Read the model definition and answer for the solid it produces. Units are mm, in the model's axes. A direction names the side the tool comes from. Give positions to 0.01 mm unless a question says otherwise; leave off trailing zeros. Order: outer loops, then holes, each group sorted by start corner. A loop starts at its lowest first (then second) coordinate and runs counter-clockwise, first axis right, second up.
Item 1: A cutting plane is placed at B-B (y = 46). Write down the section's boundary in (x, z).
Item 2: Which of the six approach directions +Z, -Z, +X, -X, +Y, -Y give full straight-line access (tool end or side, diameter ignored) to faces 1 (the face through (1.479, 44.463, -1.738)), 2 (the face through (7, 11, -9)), 3 (the face through (9, 13, -24))?
Item 3: Given pin 1 Ø1 at (x, z) = (3, -4.5) entering from -Y; pin 2 Ø4.5 at (x, z) = (11.65, -22.35) entering from +Y; pin 3 Ø1 at (y, z) = (28.5, -27.5) entering from +X, each flat-ended and moving along its own axis, determine where each tip first touches the part or whether it passes through.
Item 4: The mould has two halves that part along X. Classify faces 4 (the face through (1.48, 42.93, -34.15)), 5 (the face through (11.72, 11.52, -32.75)), 6 (the face through (0, 31, -17)): +X half, -X half, draft (parallel to the pull), parting line (faces both ways), or undercut.
Item 5: A cutting plane is placed at C-C (z = -13.6). Write down the section's boundary in (x, y), plus the area to 3 significant figures.
Item 6: A cutting plane is placed at D-D (x = 1). Write down the section's boundary in (y, z).
Item 7: A cutting plane is placed at A-A (x = 11.65). Write down the section's boundary in (y, z), plus the area to 3 significant figures.
Item 8: Find the intervals of material crossed by line 1 along X through (y, z) = (12.3, -22.35); line 2 along X through (y, z) = (53.5, -17); line 3 along Y through (x, z) = (6.25, -24), in increasing order.
from build123d import *

# Parameters (mm, degrees)
SKETCH_2_W          = 28.61033589
SKETCH_2_H          = 3
EXTRUDE_5_DEPTH     = 16
SKETCH_3_R          = 1.65
CUT_EXTRUDE_1_DEPTH = 10
SKETCH_4_R          = 1.65
SKETCH_4_R_2        = 1.25
SKETCH_4_R_3        = 9.7
EXTRUDE_8_DEPTH     = 3
FILLET_1_R          = 2


with BuildPart() as part:
    # 草图2 → 凸台-拉伸5 (new body)
    with BuildSketch(Plane.ZY):
        with Locations((-23.305167945, 11.5)):
            Rectangle(SKETCH_2_W, SKETCH_2_H)
    extrude(amount=-EXTRUDE_5_DEPTH)

    # 草图3 → 切除-拉伸1 (cut)
    with BuildSketch(Plane(origin=(0, 13, 0), x_dir=(1, 0, 0), z_dir=(0, 1, 0))):
        with Locations(Location((11.65, 31.1, 0), (0, 0, 270))):
            Circle(SKETCH_3_R)
        with Locations(Location((11.65, 22.35, 0), (0, 0, 90))):
            Circle(SKETCH_3_R)
        with Locations(Location((11.65, 13.6, 0), (0, 0, 270))):
            Circle(SKETCH_3_R)
    extrude(amount=-CUT_EXTRUDE_1_DEPTH, mode=Mode.SUBTRACT)

    # 草图4 → 凸台-拉伸8 (add)
    with BuildSketch(Plane(origin=(0, 0, 0), x_dir=(0, 0, -1), z_dir=(1, 0, 0))):
        with BuildLine():
            Line((0, 13), (37.61033589, 13))
            Line((37.61033589, 13), (37.61033589, 42.99965258))
            ThreePointArc((37.61033589, 42.99965258), (16.600372012, 63.090063758), (-2.530280254, 41.20259366))
            Line((-2.530280254, 41.20259366), (0, 13))
        make_face()
        with Locations(Location((17.49980147, 57.99965258, 0), (0, 0, 180))):
            Circle(SKETCH_4_R, mode=Mode.SUBTRACT)
        with Locations(Location((32.49980147, 42.99965258, 0), (0, 0, 180))):
            Circle(SKETCH_4_R, mode=Mode.SUBTRACT)
        with Locations(Location((17.49980147, 27.99965258, 0), (0, 0, 180))):
            Circle(SKETCH_4_R, mode=Mode.SUBTRACT)
        with Locations(Location((2.49980147, 42.99965258, 0), (0, 0, 180))):
            Circle(SKETCH_4_R, mode=Mode.SUBTRACT)
        with Locations(Location((23.354935737, 21.197394906, 0), (0, 0, 180))):
            Circle(SKETCH_4_R_2, mode=Mode.SUBTRACT)
        with Locations(Location((3.788610616, 19.472011044, 0), (0, 0, 180))):
            Circle(SKETCH_4_R, mode=Mode.SUBTRACT)
        with Locations(Location((17.49980147, 42.99965258, 0), (0, 0, 180))):
            Circle(SKETCH_4_R_3, mode=Mode.SUBTRACT)
    extrude(amount=EXTRUDE_8_DEPTH)

    # 圆角1
    fillet_1_edges = [part.edges().sort_by_distance(p)[0] for p in [
        (16, 11.5, -37.61033589),
        (1.5, 13, 0),
        (16, 11.5, -9),
    ]]
    fillet(fillet_1_edges, radius=FILLET_1_R)


solid = part.part
Response values:
1. outline: (0, -37.39) - (3, -37.39) - (3, -26.72) - (0, -26.72) - close; (0, -8.28) - (3, -8.28) - (3, 2.39) - (0, 2.39) - close
2. face 1: +X, -X
2. face 2: +Z, +X, -X, -Y
2. face 3: +Z, -Z, +X, +Y
3. pin 1: stops at y = 13
3. pin 2: stops at y = 13
3. pin 3: stops at x = 3
4. face 4: draft
4. face 5: undercut
4. face 6: -X half
5. outline: (0, 10) - (10, 10) - (10, 13) - (3, 13) - (3, 34.12) - (0, 34.12) - close; (0, 51.88) - (3, 51.88) - (3, 62.73) - (0, 62.73) - close; (13.3, 10) - (16, 10) - (16, 13) - (13.3, 13) - close
5. area: 134 mm2
6. outline: (10, -37.61) - (43, -37.61) arc R20.11 ccw (long way) to (41.2, 2.53) - (14.82, 0.16) arc R2 ccw to (13, -1.83) - (13, -9) - (10, -9) - close; hole circle Ø3.3 at (19.47, -3.79); hole circle Ø2.5 at (21.2, -23.35); hole circle Ø3.3 at (28, -17.5); hole circle Ø19.4 at (43, -17.5); hole circle Ø3.3 at (43, -32.5); hole circle Ø3.3 at (43, -2.5); hole circle Ø3.3 at (58, -17.5)
7. outline: (10, -37.61) - (13, -37.61) - (13, -32.75) - (10, -32.75) - close; (10, -29.45) - (13, -29.45) - (13, -24) - (10, -24) - close; (10, -20.7) - (13, -20.7) - (13, -15.25) - (10, -15.25) - close; (10, -11.95) - (13, -11.95) - (13, -9) - (10, -9) - close
7. area: 56.1 mm2
8. line 1: x = 0 to 10, 13.3 to 16
8. line 2: x = 0 to 3
8. line 3: y = 10 to 13
